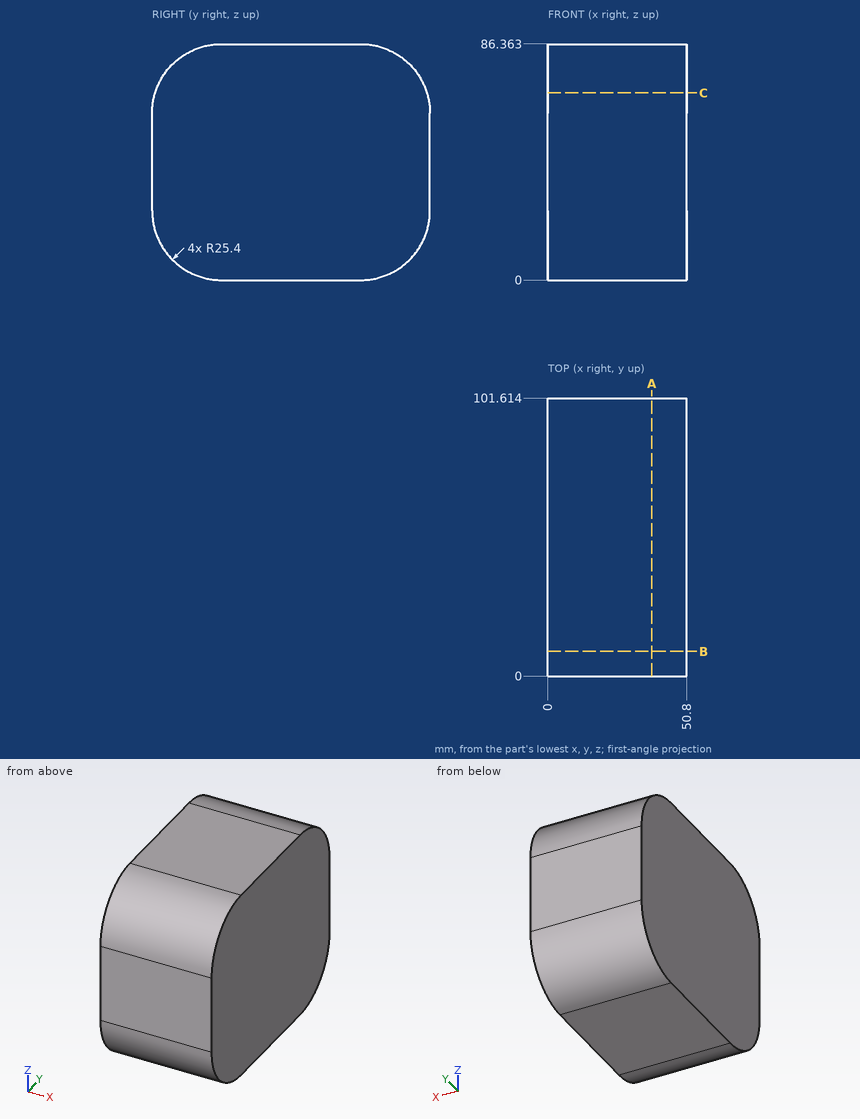
Could you check a few things on this drawing? It's one solid part, dimensions in mm from its lowest x, y, z. Round coordinates to 2 decimals unless told otherwise and drop trailing zeros. Loops run counter-clockwise (first coordinate to the right, second up) from the corner with the lowest first, then second, coordinate; pieces in that order, holes last. Notation, with made-up numbers: (60, 51) -> (117, 51) arc R23 cw to (117, 66) -> close; hole circle Ø2 at (83.5, 76.25). An arc over 180 degrees is marked (long way). One line per item, written item: value. Start each with the question number.
1. For pin 1 (3 mm diameter, centred on x = 29.5, y = 23.5, fed in from +Z); pin 2 (1.5 mm diameter, centred on x = 27, z = 15, fed in from +Y); pin 3 (5 mm diameter, centred on x = 32.5, y = 14, fed in from -Z), each with a flat end and sliding along its axis, tell me the tip position at first contact or that it passes through.
2. If we section it at A-A, the plane x = 38: Write out the boundary of the cut face in (y, z), then the cut area to 3 significant figures.
3. If we section it at C-C, the plane z = 68.5: Write out the boundary of the cut face in (x, y).
4. If I drill on probe 1 along Y at (x, z) = (38.5, 25); probe 2 along Y at (x, z) = (30, 19.5) (1 decimal); probe 3 along Z at (x, y) = (4, 9) (1 decimal), over which ranges is the centre line in solid material (lowest first)?
5. If we section it at B-B, the plane y = 9: Write out the boundary of the cut face in (x, z).
Calculated:
1. pin 1: stops at z = 86.36
1. pin 2: stops at y = 99.71
1. pin 3: stops at z = 1.61
2. outline: (0, 25.4) arc R25.4 ccw to (25.4, 0) -> (76.21, 0) arc R25.4 ccw to (101.61, 25.4) -> (101.61, 60.96) arc R25.4 ccw to (76.21, 86.36) -> (25.4, 86.36) arc R25.4 ccw to (0, 60.96) -> close
2. area: 8,220 mm²
3. outline: (0, 1.14) -> (50.8, 1.14) -> (50.8, 100.47) -> (0, 100.47) -> close
4. probe 1: y = 0 to 101.61
4. probe 2: y = 0.7 to 100.9
4. probe 3: z = 6 to 80.4
5. outline: (0, 6) -> (50.8, 6) -> (50.8, 80.36) -> (0, 80.36) -> close
